Part print with two shaded views. Sizes in mm from the minimum x, y, z corner. Give positions to 0.01 mm unless a question says otherwise; leave off trailing zeros. Write each loop counter-clockwise with the first axis right and the second up, starting at its lowest first coordinate (ties: lowest second). Pieces come first, ordered by that corner, then holes.
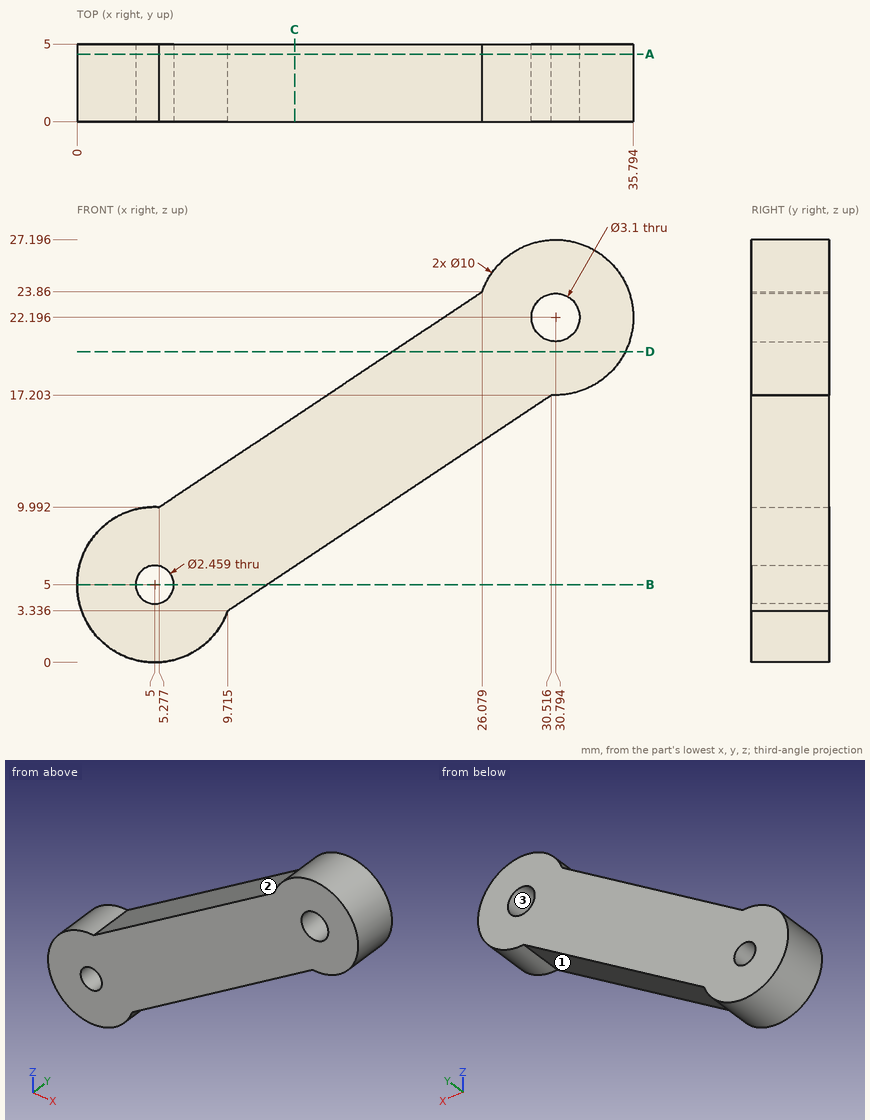
1) Saw through at B-B, the plane z = 5. Write the cut outline in (x, y).
Answers follow:
outline: (0, 0) - (3.77, 0) - (3.77, 5) - (0, 5) - close; (6.23, 0) - (12.21, 0) - (12.21, 5) - (6.23, 5) - close
2) Pin check, flat tips, straight feed: pin 1 Ø1 at (y, z) = (1.5, 23) entering from -X; pin 2 Ø2 at (x, z) = (5, 5) entering from -Y; pin 3 Ø3 at (x, y) = (20, 0.5) entering from -Z. Stop position of each tip, or through.
Answers follow:
pin 1: stops at x = 24.04
pin 2: passes through
pin 3: stops at z = 9.19
3) Wall check: L1, parallel to Z at x = 5, y = 2.9; L2, parallel to X at y = 3.8, z = 5; L3, parallel to X at y = 4.6, z = 21.75 (1 decimal). Give the ranges that are in metal, low to high.
Answers follow:
L1: z = 0 to 3.77, 6.23 to 10
L2: x = 0 to 3.77, 6.23 to 12.21
L3: x = 22.9 to 29.3, 32.3 to 35.8
4) Saw through at D-D, the plane z = 20. Write the cut outline in (x, y) (1 decimal).
Answers follow:
outline: (20.3, 0) - (35.3, 0) - (35.3, 5) - (20.3, 5) - close
5) Saw through at A-A, the plane y = 4.35. Count the separate pieces of the cut face and the enclosed holes in it.
Answers follow:
separate pieces: 1
enclosed holes: 2
6) Saw through at C-C, the plane x = 14. Write the cut outline in (y, z).
Answers follow:
outline: (0, 6.19) - (5, 6.19) - (5, 15.81) - (0, 15.81) - close
7) Two-plate mould, pull along Z, no slides. Class the marked faces 1, 2 and 3: +Z half, -Z half, draft (parallel to the pull), parting line (faces both ways), or undercut.
Answers follow:
face 1: -Z half
face 2: +Z half
face 3: undercut
